```python
from build123d import *

# Parameters (mm, degrees)
SKETCH_1_W      = 40
SKETCH_1_H      = 20
SKETCH_1_R      = 3
SKETCH_1_W_2    = 3
SKETCH_1_H_2    = 6
EXTRUDE_1_DEPTH = 1.5


with BuildPart() as part:
    # 草图1 → 凸台-拉伸1 (new body)
    with BuildSketch(Plane.XY):
        Rectangle(SKETCH_1_W, SKETCH_1_H)
        with Locations((3, 0)):
            Circle(SKETCH_1_R, mode=Mode.SUBTRACT)
        with Locations((-5, 0)):
            Rectangle(SKETCH_1_W_2, SKETCH_1_H_2, mode=Mode.SUBTRACT)
        with Locations((17, 0)):
            Rectangle(SKETCH_1_W_2, SKETCH_1_H_2, mode=Mode.SUBTRACT)
    extrude(amount=EXTRUDE_1_DEPTH)


solid = part.part
```
Work out the finished part from the listing and answer in its coordinate system (mm). A direction names the side the tool comes from. Give positions to 0.01 mm unless a question says otherwise; leave off trailing zeros. Order: outer loops, then holes, each group sorted by start corner. A loop starts at its lowest first (then second) coordinate and runs counter-clockwise, first axis right, second up. Notation, with made-up numbers: (-5, 34.25) - (36, 34.25) arc R21 cw to (36, 49.25) - close; hole circle Ø2 at (57, -8). An arc over 180 degrees is marked (long way). One line per item, written item: value. Start each with the question number.
1. This flat-tipped pin is pushed along its axis until it touches: pin 1 Ø5 at (x, y) = (3, 0) entering from -Z. Where does it stop, or does it pass through?
2. Section A-A, the plane z = 0.65 is taken. Write down the section's boundary in (x, y), then the cut area to 3 significant figures.
3. Section C-C, the plane y = 0 is taken. Write down the section's boundary in (x, z).
4. Which of the six approach directions +Z, -Z, +X, -X, +Y, -Y give full straight-line access (tool end or side, diameter ignored) to faces 4 (the face through (-5, -3, 1)), 5 (the face through (-20, 0, 1))?
5. For a pull along X with two mould halves and no side action, classify faces 1 (the face through (-3.5, 0, 1)), 2 (the face through (-0.3, 0.1, 0)), 3 (the face through (20, 0, 1)) as released by +X, released by -X, zero draft, split by the parting line, or undercut.
6. Section D-D, the plane y = 2.5 is taken. Write down the section's boundary in (x, z).
7. Consider line 1 (Y direction, x = 3, z = 0.7); line 2 (X direction, y = 2, z = 0.65); line 3 (X direction, y = 0.5, z = 0.1). Determine where each line is inside the solid, lowest interval first.
8. Section B-B, the plane x = 3 is taken. Write down the section's boundary in (y, z), then the cut area to 3 significant figures.
Filled sheet:
1. pin 1: through
2. outline: (-20, -10) - (20, -10) - (20, 10) - (-20, 10) - close; hole (-6.5, -3) - (-3.5, -3) - (-3.5, 3) - (-6.5, 3) - close; hole circle Ø6 at (3, 0); hole (15.5, -3) - (18.5, -3) - (18.5, 3) - (15.5, 3) - close
2. area: 736 mm²
3. outline: (-20, 0) - (-6.5, 0) - (-6.5, 1.5) - (-20, 1.5) - close; (-3.5, 0) - (0, 0) - (0, 1.5) - (-3.5, 1.5) - close; (6, 0) - (15.5, 0) - (15.5, 1.5) - (6, 1.5) - close; (18.5, 0) - (20, 0) - (20, 1.5) - (18.5, 1.5) - close
4. face 4: +Z, -Z
4. face 5: +Z, -Z, -X, +Y, -Y
5. face 1: undercut
5. face 2: zero draft
5. face 3: released by +X
6. outline: (-20, 0) - (-6.5, 0) - (-6.5, 1.5) - (-20, 1.5) - close; (-3.5, 0) - (1.34, 0) - (1.34, 1.5) - (-3.5, 1.5) - close; (4.66, 0) - (15.5, 0) - (15.5, 1.5) - (4.66, 1.5) - close; (18.5, 0) - (20, 0) - (20, 1.5) - (18.5, 1.5) - close
7. line 1: -10 to -3, 3 to 10
7. line 2: -20 to -6.5, -3.5 to 0.76, 5.24 to 15.5, 18.5 to 20
7. line 3: -20 to -6.5, -3.5 to 0.04, 5.96 to 15.5, 18.5 to 20
8. outline: (-10, 0) - (-3, 0) - (-3, 1.5) - (-10, 1.5) - close; (3, 0) - (10, 0) - (10, 1.5) - (3, 1.5) - close
8. area: 21.0 mm²
